The listing builds one solid part. Answer for the finished solid, in the listing's coordinates (mm). Face numbers are marked on the shaded views. A direction names the side the tool comes from. Round coordinates to 2 decimals unless told otherwise and drop trailing zeros. Order: outer loops, then holes, each group sorted by start corner. A loop starts at its lowest first (then second) coordinate and runs counter-clockwise, first axis right, second up. Notation, with made-up numbers: M -37.75,67.5 L -5.75,67.5 A19 cw -5.75,100.5 Z; hole C 62,-17.75 d11. An arc over 180 degrees is marked long. Write item = value, one per line. Start each with the question number.
(1) Straight lines are drawn through the part: probe 1 along Y at (x, z) = (0.8, 25.5); probe 2 along X at (y, z) = (-0.1, 22.5); probe 3 along Z at (x, y) = (1.75, -0.95). For each, find the intervals that lie inside material, in ascending order. Write a range as from..to.
(2) A cutting plane is placed at A-A, the plane x = 0. Determine the outline of the cut face in (y, z), and give its area (3 significant figures).
(3) Each of these flat-tipped pins is pushed along its axis until it touches: pin 1 (0.9 mm diameter, centred on x = 0.5, z = 19, fed in from -Y); pin 2 (0.9 mm diameter, centred on x = 0.5, z = 24.5, fed in from +Y); pin 3 (1.3 mm diameter, centred on y = 0, z = 1.5, fed in from +X). Where does it stop, or does it pass through?
(4) Which of the six approach directions +Z, -Z, +X, -X, +Y, -Y give full straight-line access (tool end or side, diameter ignored) to the marked faces 1, 2, 3, 4 and 5?
(5) A cutting plane is placed at D-D, the plane z = 23.5. Determine the outline of the cut face in (x, y), and give its area (3 significant figures).
(6) A cutting plane is placed at B-B, the plane y = -0.7. Determine the outline of the cut face in (x, z).
(7) A cutting plane is placed at C-C, the plane z = 2.75. Determine the outline of the cut face in (x, y).
from build123d import *

# Parameters (mm, degrees)
SKETCH1_R               = 2.5
BOSS_EXTRUDE1_DEPTH     = 28.879
SKETCH2_R               = 2.5
CUT_EXTRUDE1_DEPTH      = 5
CUT_EXTRUDE2_DEPTH      = 15.879
CUT_EXTRUDE3_DEPTH      = 3.5
CUT_EXTRUDE3_DEPTH_BACK = 3.5


with BuildPart() as part:
    # Sketch1 → Boss-Extrude1 (new body)
    with BuildSketch(Plane.XY):
        Circle(SKETCH1_R)
    extrude(amount=BOSS_EXTRUDE1_DEPTH)

    # Sketch2 → Cut-Extrude1 (cut)
    with BuildSketch(Plane(origin=(0, 0, 0), x_dir=(-1, 0, 0), z_dir=(0, 0, -1))):
        Circle(SKETCH2_R)
        with BuildLine():
            Line((-1.5, 1.322875656), (-1.5, -1.322875656))
            ThreePointArc((-1.5, -1.322875656), (0, -2), (1.5, -1.322875656))
            Line((1.5, -1.322875656), (1.5, 1.322875656))
            ThreePointArc((1.5, 1.322875656), (0, 2), (-1.5, 1.322875656))
        make_face(mode=Mode.SUBTRACT)
    extrude(amount=-CUT_EXTRUDE1_DEPTH, mode=Mode.SUBTRACT)

    # Sketch3 → Cut-Extrude2 (cut)
    with BuildSketch(Plane.XY.offset(28.879)):
        with BuildLine():
            Line((-1.5, 2), (1.5, 2))
            ThreePointArc((1.5, 2), (0, 2.5), (-1.5, 2))
        make_face()
        with BuildLine():
            Line((-1.5, -2), (1.5, -2))
            ThreePointArc((1.5, -2), (0, -2.5), (-1.5, -2))
        make_face()
    extrude(amount=-CUT_EXTRUDE2_DEPTH, mode=Mode.SUBTRACT)

    # Sketch4 → Cut-Extrude3 (cut, two sides)
    with BuildSketch(Plane(origin=(0, 0, 0), x_dir=(0, 0, -1), z_dir=(1, 0, 0))) as cut_extrude3_sk:
        with BuildLine():
            Line((-13, 2.5), (-13, 2))
            ThreePointArc((-13, 2), (-12.646446609, 2.146446609), (-12.5, 2.5))
            Line((-12.5, 2.5), (-13, 2.5))
        make_face()
        with BuildLine():
            Line((-13, -2.5), (-13, -2))
            ThreePointArc((-13, -2), (-12.646446609, -2.146446609), (-12.5, -2.5))
            Line((-12.5, -2.5), (-13, -2.5))
        make_face()
    extrude(amount=CUT_EXTRUDE3_DEPTH, mode=Mode.SUBTRACT)
    extrude(cut_extrude3_sk.sketch, amount=-CUT_EXTRUDE3_DEPTH_BACK, mode=Mode.SUBTRACT)


solid = part.part
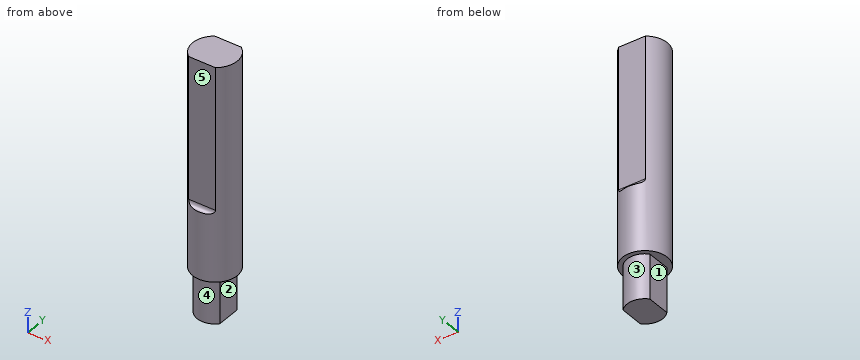
Reported:
q1.probe_1 = -2..2
q1.probe_2 = -2.5..2.5
q1.probe_3 = 5..28.88
q2.outline = M -2.5,5 L -2,5 L -2,0 L 2,0 L 2,5 L 2.5,5 L 2.5,12.5 A0.5 cw 2,13 L 2,28.88 L -2,28.88 L -2,13 A0.5 cw -2.5,12.5 Z
q2.area = 123 mm²
q3.pin_1 = -2
q3.pin_2 = 2
q3.pin_3 = 1.5
q4.face_1 = -Z, -X, +Y, -Y
q4.face_2 = -Z, +X, +Y, -Y
q4.face_3 = -Z, +Y
q4.face_4 = -Z, -Y
q4.face_5 = +Z, +X, -X, -Y
q5.outline = M -1.5,-2 L 1.5,-2 A2.5 ccw 1.5,2 L -1.5,2 A2.5 ccw Z
q5.area = 17.6 mm²
q6.outline = M -2.4,5 L -1.5,5 L -1.5,0 L 1.5,0 L 1.5,5 L 2.4,5 L 2.4,28.88 L -2.4,28.88 Z
q7.outline = M -1.5,-1.32 A2 ccw 1.5,-1.32 L 1.5,1.32 A2 ccw -1.5,1.32 Z
